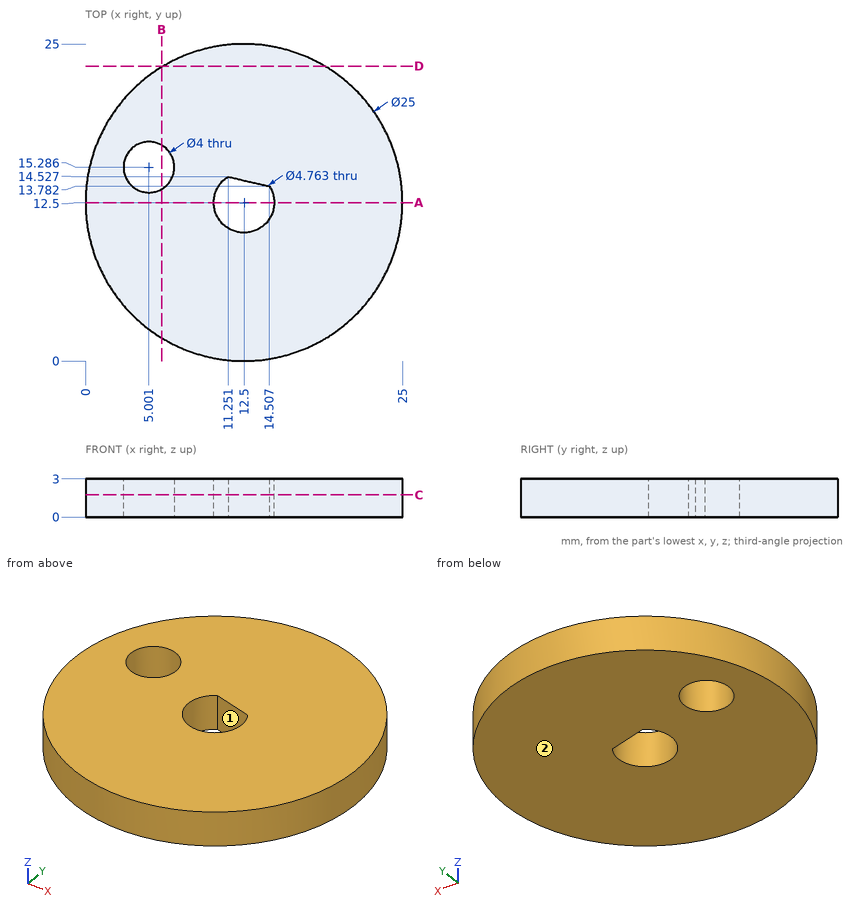
Input: dimensioned drawing with shaded views. Units: mm. Origin: part minimum x, y, z. A direction names the side the tool comes from. Give positions to 0.01 mm unless a question says otherwise; leave off trailing zeros. Write each loop counter-clockwise with the first axis right and the second up, starting at its lowest first coordinate (ties: lowest second). Pieces come first, ordered by that corner, then holes. Notation, with made-up numbers: (89.25, 66) - (111.25, 66) arc R11 ccw to (111.25, 81) - close; hole circle Ø6 at (56, 42.5). An arc over 180 degrees is marked (long way). One line per item, written item: value. Start each with the question number.
Q1. First-contact query: pin 1 Ø5 at (x, y) = (20, 11) entering from -Z; pin 2 Ø3 at (x, y) = (12.5, 12.5) entering from -Z. Flat tips, straight axial feed; report the tip coordinate or a pass-through.
Q2. Section query C-C, the plane z = 1.75. Return the cut outline in (x, y), then the cut area to 3 significant figures.
Q3. Section query B-B, the plane x = 6. Return the cut outline in (y, z).
Q4. Section query D-D, the plane y = 23.25. Return the cut outline in (x, z).
Q5. Set-up query: the marked faces 1 and 2. Return all of +Z, -Z, +X, -X, +Y, -Y with unobstructed straight access to the full face (end or side cutting, diameter ignored); none if empty.
Q6. Material intervals for probe 1 along X at (y, z) = (12.25, 0.95); probe 2 along Y at (x, z) = (12.5, 2.3); probe 3 along X at (y, z) = (15.25, 0.2) (1 decimal), sorted ascending. Write a range as from..to.
Q7. Section query A-A, the plane y = 12.5. Return the cut outline in (x, z).
Answer:
1. pin 1: stops at z = 0
1. pin 2: passes through
2. outline: circle Ø25 at (12.5, 12.5); hole circle Ø4 at (5, 15.29); hole (11.25, 14.53) arc R2.38 ccw (long way) to (14.51, 13.78) - close
2. area: 462 mm2
3. outline: (1.82, 0) - (13.55, 0) - (13.55, 3) - (1.82, 3) - close; (17.02, 0) - (23.18, 0) - (23.18, 3) - (17.02, 3) - close
4. outline: (6.12, 0) - (18.88, 0) - (18.88, 3) - (6.12, 3) - close
5. face 1: +Z, -Z
5. face 2: -Z, +X, -X, +Y, -Y
6. probe 1: x = 0..10.13, 14.87..25
6. probe 2: y = 0..10.12, 14.24..25
6. probe 3: x = 0.3..3, 7..24.7
7. outline: (0, 0) - (10.12, 0) - (10.12, 3) - (0, 3) - close; (14.88, 0) - (25, 0) - (25, 3) - (14.88, 3) - close
